The listing builds one solid part. Answer for the finished solid, in the listing's coordinates (mm). Face numbers are marked on the shaded views. A direction names the side the tool comes from. Give positions to 0.01 mm unless a question says otherwise; leave off trailing zeros. Loops run counter-clockwise (first coordinate to the right, second up) from the corner with the lowest first, then second, coordinate; pieces in that order, holes last.
Item 1: Section C-C, the plane z = 10 is taken. Give the vertices of the cut face in (x, y).
Item 2: Section A-A, the plane z = 5.75 is taken. Give the vertices of the cut face in (x, y).
Item 3: Section B-B, the plane z = 3 is taken. Give the vertices of the cut face in (x, y).
Item 4: Consider line 1 along Y through (x, z) = (0, 4.75); line 2 along Z through (x, y) = (1, -4.25); line 3 along Y through (x, z) = (1.5, 11). Determine where each line is inside the solid, lowest interval first.
Item 5: Each of these flat-tipped pins is pushed along its axis until it touches: pin 1 Ø3.5 at (y, z) = (5, 8.5) entering from -X; pin 2 Ø1 at (x, z) = (6, 9) entering from -Y; pin 3 Ø7.5 at (x, y) = (0, 0) entering from +Z; pin 4 Ø5 at (x, z) = (6, 6) entering from -Y. Where does it stop, or does it pass through?
Item 6: A tool of negligible diameter and unlimited length cuts with its end or side. For the marked faces 4, 5, 6 and 7, from which of +Z, -Z, +X, -X, +Y, -Y can it reach the whole face along a straight path? Write none if from no direction.
Item 7: The mould has two halves that part along X. Classify the marked faces 1, 2 and 3: pulls with the +X half, pulls with the -X half, needs draft (parallel to the pull), parting line crosses it, or undercut.
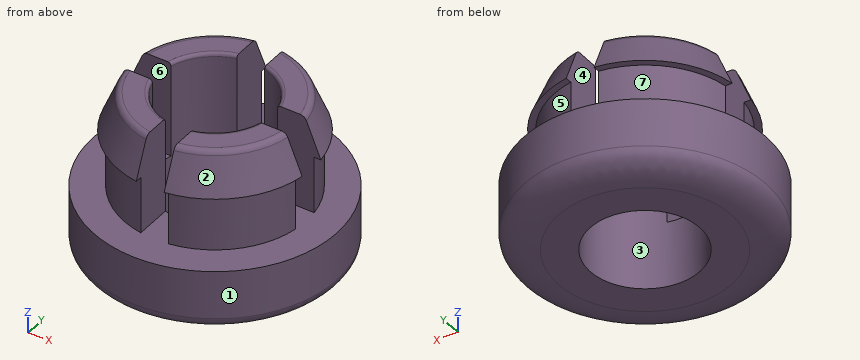
from build123d import *

# Parameters (mm, degrees)
F2_W     = 2.1
F2_H     = 6.45
F2_W_2   = 6.45
F2_H_2   = 2.1
F3_DEPTH = 7.2
F4_R     = 0.25
F5_R     = 0.5


with BuildPart() as f1:
    # F0 (on Front) → F1 (revolve)
    with BuildSketch(Plane.XZ):
        with BuildLine():
            Line((4.15, 12.2), (4.15, 0))
            Line((4.15, 0), (6.55, 0))
            add(Edge.make_bspline(
                [(6.55, 0), (7.5164148551, 0), (9.15, 0.4540091534), (9.15, 1.3436317709)],
                knots=[0, 0, 0, 0, 2.926661295, 2.926661295, 2.926661295, 2.926661295], degree=3))
            Line((9.15, 1.3436317709), (9.15, 5))
            Line((9.15, 5), (6.85, 5))
            Line((6.85, 5), (6.85, 9.3))
            Line((6.85, 9.3), (7.35, 9.3))
            Line((7.35, 9.3), (6.15, 12.2))
            Line((6.15, 12.2), (4.15, 12.2))
        make_face()
    revolve(axis=Axis((0, 0, 4.5666272921), (0, 0, 1)))

    # F2 (on face) → F3 (cut)
    with BuildSketch(Plane.XY.offset(12.2)):
        with Locations((0, 4.275)):
            Rectangle(F2_W, F2_H)
        with Locations((4.275, 0)):
            Rectangle(F2_W_2, F2_H_2)
        Rectangle(F2_W, F2_H_2)
        with Locations((0, -4.275)):
            Rectangle(F2_W, F2_H)
        with Locations((-4.275, 0)):
            Rectangle(F2_W_2, F2_H_2)
    extrude(amount=-F3_DEPTH, mode=Mode.SUBTRACT)

    # F4
    f4_edges = [f1.edges().sort_by_distance(p)[0] for p in [
        (-2.934493, -2.934493, 12.2),
        (-2.934493, 2.934493, 12.2),
        (2.934493, 2.934493, 12.2),
        (2.934493, -2.934493, 12.2),
    ]]
    fillet(f4_edges, radius=F4_R)

    # F5
    f5_edges = [f1.edges().sort_by_distance(p)[0] for p in [
        (4.348707, 4.348707, 12.2),
        (-4.348707, 4.348707, 12.2),
        (-4.348707, -4.348707, 12.2),
        (4.348707, -4.348707, 12.2),
    ]]
    fillet(f5_edges, radius=F5_R)


solid = f1.part
Worked answers:
1. outline: (-6.98, -1.05) arc R7.06 ccw to (-1.05, -6.98) - (-1.05, -4.01) arc R4.15 cw to (-4.01, -1.05) - close; (-6.98, 1.05) - (-4.01, 1.05) arc R4.15 cw to (-1.05, 4.01) - (-1.05, 6.98) arc R7.06 ccw to start; (1.05, -6.98) arc R7.06 ccw to (6.98, -1.05) - (4.01, -1.05) arc R4.15 cw to (1.05, -4.01) - close; (1.05, 4.01) arc R4.15 cw to (4.01, 1.05) - (6.98, 1.05) arc R7.06 ccw to (1.05, 6.98) - close
2. outline: (-6.77, -1.05) arc R6.85 ccw to (-1.05, -6.77) - (-1.05, -4.01) arc R4.15 cw to (-4.01, -1.05) - close; (-6.77, 1.05) - (-4.01, 1.05) arc R4.15 cw to (-1.05, 4.01) - (-1.05, 6.77) arc R6.85 ccw to start; (1.05, -6.77) arc R6.85 ccw to (6.77, -1.05) - (4.01, -1.05) arc R4.15 cw to (1.05, -4.01) - close; (1.05, 4.01) arc R4.15 cw to (4.01, 1.05) - (6.77, 1.05) arc R6.85 ccw to (1.05, 6.77) - close
3. outline: circle Ø18.3 at (0, 0); hole circle Ø8.3 at (0, 0)
4. line 1: y = -9.15 to -4.15, 4.15 to 9.15
4. line 2: z = 0 to 5
4. line 3: y = -6.48 to -3.87, 3.87 to 6.48
5. pin 1: stops at x = -6.49
5. pin 2: stops at y = -4.76
5. pin 3: passes through
5. pin 4: stops at y = -8.36
6. face 4: +Z, +Y, -Y
6. face 5: +X, +Y
6. face 6: +Z, +X, -X
6. face 7: -X, +Y
7. face 1: parting line crosses it
7. face 2: pulls with the +X half
7. face 3: undercut
